```python
from build123d import *

# Parameters (mm, degrees)
SKETCH1_R           = 27.2415
BOSS_EXTRUDE1_DEPTH = 3.175
SKETCH2_R           = 25.3365
BOSS_EXTRUDE2_DEPTH = 3.175
SKETCH5_R           = 4.2037
CUT_EXTRUDE1_DEPTH  = 6.35
CUT_EXTRUDE2_REACH  = 8.35
SKETCH6_R           = 4.5085
CUT_EXTRUDE3_REACH  = 8.35
SKETCH9_R           = 1.016


with BuildPart() as part:
    # Sketch1 → Boss-Extrude1 (new body)
    with BuildSketch(Plane(origin=(0, 0, 0), x_dir=(1, 0, 0), z_dir=(0, 1, 0))):
        Circle(SKETCH1_R)
    extrude(amount=BOSS_EXTRUDE1_DEPTH)

    # Sketch2 → Boss-Extrude2 (add)
    with BuildSketch(Plane(origin=(0, 3.175, 0), x_dir=(1, 0, 0), z_dir=(0, 1, 0))):
        Circle(SKETCH2_R)
    extrude(amount=BOSS_EXTRUDE2_DEPTH)

    # Sketch5 → Cut-Extrude1 (cut)
    with BuildSketch(Plane.XZ):
        with Locations((-12.992582175, -1.862973623)):
            Circle(SKETCH5_R)
    extrude(amount=-CUT_EXTRUDE1_DEPTH, mode=Mode.SUBTRACT)

    # Sketch6 → Cut-Extrude2 (cut, up to next)
    with BuildSketch(Plane.XZ, mode=Mode.PRIVATE) as cut_extrude2_sk1:
        Circle(SKETCH6_R)
    cut_extrude2_tool1 = extrude(cut_extrude2_sk1.sketch, amount=-CUT_EXTRUDE2_REACH, mode=Mode.PRIVATE) & part.part
    add(cut_extrude2_tool1.solids().sort_by_distance((0, 0, 0))[0], mode=Mode.SUBTRACT)

    # Sketch9 → Cut-Extrude3 (cut, up to next)
    with BuildSketch(Plane(origin=(0, 6.35, 0), x_dir=(1, 0, 0), z_dir=(0, 1, 0)), mode=Mode.PRIVATE) as cut_extrude3_sk1:
        with Locations((13.97, 5.715)):
            Circle(SKETCH9_R)
    cut_extrude3_tool1 = extrude(cut_extrude3_sk1.sketch, amount=-CUT_EXTRUDE3_REACH, mode=Mode.PRIVATE) & part.part
    add(cut_extrude3_tool1.solids().sort_by_distance((13.97, 6.35, -5.715))[0], mode=Mode.SUBTRACT)
    # Sketch9 → Cut-Extrude3 (cut, up to next)
    with BuildSketch(Plane(origin=(0, 6.35, 0), x_dir=(1, 0, 0), z_dir=(0, 1, 0)), mode=Mode.PRIVATE) as cut_extrude3_sk2:
        with Locations((13.97, 1.905)):
            Circle(SKETCH9_R)
    cut_extrude3_tool2 = extrude(cut_extrude3_sk2.sketch, amount=-CUT_EXTRUDE3_REACH, mode=Mode.PRIVATE) & part.part
    add(cut_extrude3_tool2.solids().sort_by_distance((13.97, 6.35, -1.905))[0], mode=Mode.SUBTRACT)
    # Sketch9 → Cut-Extrude3 (cut, up to next)
    with BuildSketch(Plane(origin=(0, 6.35, 0), x_dir=(1, 0, 0), z_dir=(0, 1, 0)), mode=Mode.PRIVATE) as cut_extrude3_sk3:
        with Locations((13.97, -1.905)):
            Circle(SKETCH9_R)
    cut_extrude3_tool3 = extrude(cut_extrude3_sk3.sketch, amount=-CUT_EXTRUDE3_REACH, mode=Mode.PRIVATE) & part.part
    add(cut_extrude3_tool3.solids().sort_by_distance((13.97, 6.35, 1.905))[0], mode=Mode.SUBTRACT)
    # Sketch9 → Cut-Extrude3 (cut, up to next)
    with BuildSketch(Plane(origin=(0, 6.35, 0), x_dir=(1, 0, 0), z_dir=(0, 1, 0)), mode=Mode.PRIVATE) as cut_extrude3_sk4:
        with Locations((13.97, -5.715)):
            Circle(SKETCH9_R)
    cut_extrude3_tool4 = extrude(cut_extrude3_sk4.sketch, amount=-CUT_EXTRUDE3_REACH, mode=Mode.PRIVATE) & part.part
    add(cut_extrude3_tool4.solids().sort_by_distance((13.97, 6.35, 5.715))[0], mode=Mode.SUBTRACT)


solid = part.part
```
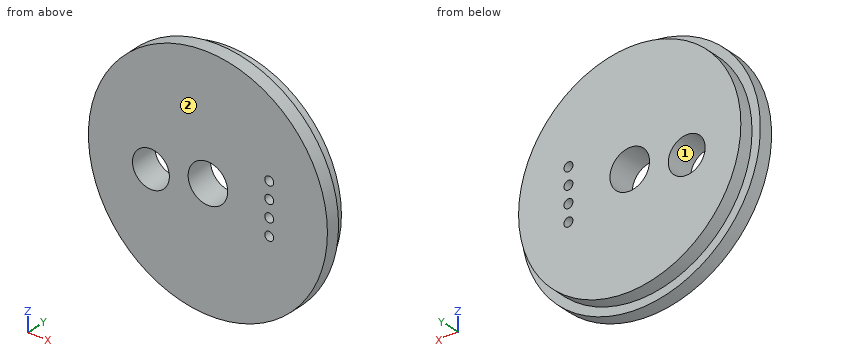
Geometry: final body of the model. Coordinates: model frame, mm. Face numbers are marked on the shaded views. Round coordinates to 2 decimals unless told otherwise and drop trailing zeros. Loops run counter-clockwise (first coordinate to the right, second up) from the corner with the lowest first, then second, coordinate; pieces in that order, holes last. Notation, with made-up numbers: (-0.75, 20.25) -> (32.25, 20.25) arc R12 cw to (32.25, 39.25) -> close; hole circle Ø3 at (21.25, 67). An arc over 180 degrees is marked (long way). Use one line per item in the form item = value.
Item 1: Cut plane A-A on z = 0. Give the number of separate pieces and of enclosed holes in the cut face, then the cut area to 3 significant figures.
Evaluation:
separate_pieces = 3
enclosed_holes = 0
area = 229 mm2
Item 2: Contact query for flat-ended pins moving along their axis: pin 1 Ø5 at (x, z) = (-15.5, 10.5) entering from -Y; pin 2 Ø1.8 at (x, z) = (13.97, 5.715) entering from -Y; pin 3 Ø2 at (x, y) = (-10.5, 2) entering from +Z. Output: stop coordinate, or through.
Evaluation:
pin_1 = 0
pin_2 = through
pin_3 = 25.53
Item 3: Cut plane C-C on y = 1.5. Output: boundary loops of the cut face in (x, z) (1 decimal).
Evaluation:
outline = circle Ø54.5 at (0, 0); hole circle Ø8.4 at (-13, -1.9); hole circle Ø9 at (0, 0); hole circle Ø2 at (14, -5.7); hole circle Ø2 at (14, -1.9); hole circle Ø2 at (14, 1.9); hole circle Ø2 at (14, 5.7)
Item 4: Material intervals for probe 1 along Z at (x, y) = (13.97, 1.5); probe 2 along Z at (x, y) = (13.97, 4); probe 3 along X at (y, z) = (5.25, -5), sorted ascending.
Evaluation:
probe_1 = -23.39 to -6.73, -4.7 to -2.92, -0.89 to 0.89, 2.92 to 4.7, 6.73 to 23.39
probe_2 = -21.14 to -6.73, -4.7 to -2.92, -0.89 to 0.89, 2.92 to 4.7, 6.73 to 21.14
probe_3 = -24.84 to -15.79, -10.19 to 13.25, 14.69 to 24.84
Item 5: Draft query along X for the marked faces 1 and 2. Return one class per face: released by +X, released by -X, zero draft, split by the parting line, or undercut.
Evaluation:
face_1 = undercut
face_2 = zero draft
Item 6: Cut plane D-D on x = 13.97. Output: boundary loops of the cut face in (y, z) (3 decimals), then the cut area to 3 significant figures.
Evaluation:
outline = (0, -23.387) -> (3.175, -23.387) -> (3.175, -21.137) -> (6.35, -21.137) -> (6.35, -6.731) -> (0, -6.731) -> close; (0, -4.699) -> (6.35, -4.699) -> (6.35, -2.921) -> (0, -2.921) -> close; (0, -0.889) -> (6.35, -0.889) -> (6.35, 0.889) -> (0, 0.889) -> close; (0, 2.921) -> (6.35, 2.921) -> (6.35, 4.699) -> (0, 4.699) -> close; (0, 6.731) -> (6.35, 6.731) -> (6.35, 21.137) -> (3.175, 21.137) -> (3.175, 23.387) -> (0, 23.387) -> close
area = 231 mm2
Item 7: Cut plane B-B on x = -13.5. Output: boundary loops of the cut face in (y, z) (3 decimals).
Evaluation:
outline = (0, -23.661) -> (3.175, -23.661) -> (3.175, -21.44) -> (6.35, -21.44) -> (6.35, -6.036) -> (0, -6.036) -> close; (0, 2.31) -> (6.35, 2.31) -> (6.35, 21.44) -> (3.175, 21.44) -> (3.175, 23.661) -> (0, 23.661) -> close
